```python
from build123d import *

# Parameters (mm, degrees)
SKETCH1_R           = 11.1125
SKETCH1_R_2         = 2.5527
BOSS_EXTRUDE1_DEPTH = 2.54


with BuildPart() as part:
    # Sketch1 → Boss-Extrude1 (new body)
    with BuildSketch(Plane(origin=(0, 0, 0), x_dir=(1, 0, 0), z_dir=(0, 1, 0))):
        with BuildLine():
            Line((-40.775, -27.44), (-40.775, 27.44))
            ThreePointArc((-40.775, 27.44), (-39.659076836, 30.134076836), (-36.965, 31.25))
            Line((-36.965, 31.25), (-15.375, 31.25))
            ThreePointArc((-15.375, 31.25), (-14.228907316, 31.073534307), (-13.188980532, 30.560483758))
            Line((-13.188980532, 30.560483758), (10.019255896, 14.302217225))
            ThreePointArc((10.019255896, 14.302217225), (17.4625, 0), (10.019255896, -14.302217225))
            Line((10.019255896, -14.302217225), (-13.188980532, -30.560483758))
            ThreePointArc((-13.188980532, -30.560483758), (-14.228907316, -31.073534307), (-15.375, -31.25))
            Line((-15.375, -31.25), (-36.965, -31.25))
            ThreePointArc((-36.965, -31.25), (-39.659076836, -30.134076836), (-40.775, -27.44))
        make_face()
        with Locations(Location((0, 0, 0), (0, 0, 270))):
            Circle(SKETCH1_R, mode=Mode.SUBTRACT)
        with Locations(Location((-28.075, 25.4, 0), (0, 0, 270))):
            Circle(SKETCH1_R_2, mode=Mode.SUBTRACT)
        with Locations(Location((-28.075, 12.7, 0), (0, 0, 270))):
            Circle(SKETCH1_R_2, mode=Mode.SUBTRACT)
        with Locations(Location((-28.075, 0, 0), (0, 0, 270))):
            Circle(SKETCH1_R_2, mode=Mode.SUBTRACT)
        with Locations(Location((-28.075, -12.7, 0), (0, 0, 270))):
            Circle(SKETCH1_R_2, mode=Mode.SUBTRACT)
        with Locations(Location((-28.075, -25.4, 0), (0, 0, 270))):
            Circle(SKETCH1_R_2, mode=Mode.SUBTRACT)
    extrude(amount=BOSS_EXTRUDE1_DEPTH)


solid = part.part
```
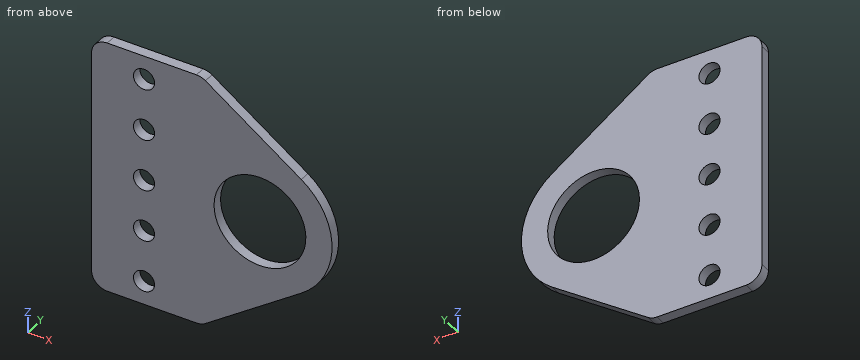
The listing builds one solid part. Answer for the finished solid, in the listing's coordinates (mm). Coordinates: 2 decimals unless noted, no trailing zeros. Write each loop counter-clockwise with the first axis right and the second up, starting at its lowest first coordinate (ties: lowest second). Pieces come first, ordered by that corner, then holes. Notation, with made-up numbers: M 34.5,21.5 L 46.5,21.5 A27 cw 46.5,42.5 Z; hole C -34,-34.5 d8. An arc over 180 degrees is marked long. Use a Markdown table: item, result. Add a question column.
1. Section A-A (z = 0) is taken. Give the vertices of the cut face in (x, y) (1 decimal).
2. Section D-D (y = 0.4) is taken. Count the separate pieces of the cut face and the enclosed holes in it, plus the area to 3 significant figures.
3. Given P1, Ø18, axis at x = 0, z = 0, coming from the +Y side; P2, Ø1.5, axis at x = -14.5, y = 0.5, coming from the +Z side; P3, Ø1, axis at y = 1.5, z = 12, coming from the +X side, each flat-ended and moving along its own axis, determine where each tip first touches the part or whether it passes through.
4. Section C-C (x = -2.5) is taken. Give the vertices of the cut face in (y, z).
5. Section B-B (z = -8) is taken. Give the vertices of the cut face in (x, y) (3 decimals).
6. Straight lines are drawn through the part: line 1 along X through (y, z) = (1.25, 1) (3 decimals); line 2 along Z through (x, y) = (-26, 0.7); line 3 along X through (y, z) = (1.85, 25.4) (3 decimals). For each, find the intervals that lie inside material, in ascending order. Write a range as [from, to].
Data:
| question | item | result |
|---|---|---|
| 1 | outline | M -40.8,0 L -30.6,0 L -30.6,2.5 L -40.8,2.5 Z; M -25.5,0 L -11.1,0 L -11.1,2.5 L -25.5,2.5 Z; M 11.1,0 L 17.5,0 L 17.5,2.5 L 11.1,2.5 Z |
| 2 | separate pieces | 1 |
| 2 | enclosed holes | 6 |
| 2 | area | 2,420 mm2 |
| 3 | P1 | passes through |
| 3 | P2 | stops at z = 31.25 |
| 3 | P3 | stops at x = 13.14 |
| 4 | outline | M 0,-23.07 L 2.54,-23.07 L 2.54,-10.83 L 0,-10.83 Z; M 0,10.83 L 2.54,10.83 L 2.54,23.07 L 0,23.07 Z |
| 5 | outline | M -40.775,0 L -7.713,0 L -7.713,2.54 L -40.775,2.54 Z; M 7.713,0 L 15.522,0 L 15.522,2.54 L 7.713,2.54 Z |
| 6 | line 1 | x = [-40.775, -30.424], [-25.726, -11.067], [11.067, 17.434] |
| 6 | line 2 | z = [-31.25, -26.89], [-23.91, -14.19], [-11.21, -1.49], [1.49, 11.21], [14.19, 23.91], [26.89, 31.25] |
| 6 | line 3 | x = [-40.775, -30.628], [-25.522, -5.823] |
